Geometry check sheet. Reference: the model listing, model coordinates, mm. Coordinates: 2 decimals unless noted, no trailing zeros. Loops run counter-clockwise (first coordinate to the right, second up) from the corner with the lowest first, then second, coordinate; pieces in that order, holes last. Notation, with made-up numbers: M 27,27 L 39,27 A14 ccw 39,35 Z; hole C 25,53.5 d3. An arc over 180 degrees is marked long. Use CSV: the item, a comma, the result in double quotes.
```python
from build123d import *

# Parameters (mm, degrees)
SKETCH1_R           = 7
BOSS_EXTRUDE1_DEPTH = 5
SKETCH2_R           = 7.5
CUT_EXTRUDE1_DEPTH  = 10


with BuildPart() as part:
    # Sketch1 → Boss-Extrude1 (new body)
    with BuildSketch(Plane(origin=(0, 0, 0), x_dir=(1, 0, 0), z_dir=(0, 1, 0))):
        with BuildLine():
            Line((-415.542365302, 422.631578947), (-351.296475424, 422.631578947))
            Line((-351.296475424, 422.631578947), (-351.296475424, 222.631578947))
            Line((-351.296475424, 222.631578947), (-415.542365302, 222.631578947))
            Line((-415.542365302, 222.631578947), (-449.708642176, 172.131578947))
            Line((-449.708642176, 172.131578947), (-449.708642176, 121.631578947))
            ThreePointArc((-449.708642176, 121.631578947), (-452.637574364, 114.560511136), (-459.708642176, 111.631578947))
            Line((-459.708642176, 111.631578947), (-479.708642176, 111.631578947))
            ThreePointArc((-479.708642176, 111.631578947), (-486.779709988, 114.560511136), (-489.708642176, 121.631578947))
            Line((-489.708642176, 121.631578947), (-489.708642176, 172.131578947))
            Line((-489.708642176, 172.131578947), (-524.868977384, 222.631578947))
            Line((-524.868977384, 222.631578947), (-691.296475424, 222.631578947))
            Line((-691.296475424, 222.631578947), (-691.296475424, 142.631578947))
            Line((-691.296475424, 142.631578947), (-1821.296475424, 142.631578947))
            Line((-1821.296475424, 142.631578947), (-1821.296475424, 502.631578947))
            Line((-1821.296475424, 502.631578947), (-691.296475424, 502.631578947))
            Line((-691.296475424, 502.631578947), (-691.296475424, 422.631578947))
            Line((-691.296475424, 422.631578947), (-524.868977384, 422.631578947))
            Line((-524.868977384, 422.631578947), (-489.708642176, 473.131578947))
            Line((-489.708642176, 473.131578947), (-489.708642176, 523.631578947))
            ThreePointArc((-489.708642176, 523.631578947), (-486.779709988, 530.702646759), (-479.708642176, 533.631578947))
            Line((-479.708642176, 533.631578947), (-459.708642176, 533.631578947))
            ThreePointArc((-459.708642176, 533.631578947), (-452.637574364, 530.702646759), (-449.708642176, 523.631578947))
            Line((-449.708642176, 523.631578947), (-449.708642176, 473.131578947))
            Line((-449.708642176, 473.131578947), (-415.542365302, 422.631578947))
        make_face()
        with Locations((-469.708642176, 492.631578947)):
            Circle(SKETCH1_R, mode=Mode.SUBTRACT)
        with Locations((-469.708642176, 152.631578947)):
            Circle(SKETCH1_R, mode=Mode.SUBTRACT)
    extrude(amount=BOSS_EXTRUDE1_DEPTH)

    # Sketch2 → Cut-Extrude1 (cut)
    with BuildSketch(Plane(origin=(0, 5, 0), x_dir=(1, 0, 0), z_dir=(0, 1, 0))):
        with Locations((-1597.770206395, 392.549644623)):
            Circle(SKETCH2_R)
        with Locations((-1597.770206395, 240.60770245)):
            Circle(SKETCH2_R)
    extrude(amount=-CUT_EXTRUDE1_DEPTH, mode=Mode.SUBTRACT)


solid = part.part
```
1. Section check D-D, the plane z = -205.5. Record the cut outline in (x, y), plus the area to 3 significant figures.
The answers:
outline,"M -1821.3,0 L -691.3,0 L -691.3,5 L -1821.3,5 Z; M -512.94,0 L -427.13,0 L -427.13,5 L -512.94,5 Z"
area,"6,080 mm^2"
2. Gauge pin test, flat ends, axial feed: P1, Ø1.5, axis at x = -1157, y = 2, coming from the -Z side; P2, Ø11, axis at x = -469.71, z = -152.63, coming from the +Y side; P3, Ø3, axis at x = -528, y = 3.5, coming from the -Z side; P4, Ø2.5, axis at y = 2.5, z = -154, coming from the +X side. Record the tip position at first contact, or that the pin passes through.
The answers:
P1,"z = -502.63"
P2,"through"
P3,"z = -422.63"
P4,"x = -449.71"
3. Section check A-A, the plane z = -454.5. Record the cut outline in (x, y), plus the area to 3 significant figures.
The answers:
outline,"M -1821.3,0 L -691.3,0 L -691.3,5 L -1821.3,5 Z; M -502.68,0 L -437.1,0 L -437.1,5 L -502.68,5 Z"
area,"5,980 mm^2"
4. Thickness scan on line 1 (Z direction, x = -1700, y = 2.7); line 2 (Z direction, x = -571.5, y = 4.3); line 3 (X direction, y = 3.7, z = -438.5). Record the ranges inside material, lowest first. Write a range as [from, to].
The answers:
line 1,"[-502.63, -142.63]"
line 2,"[-422.63, -222.63]"
line 3,"[-1821.3, -691.3], [-513.82, -426.28]"
5. Release check for a two-part mould opening along X. For faces 1 (the flat face through (-507.535, 2.465, -447.528)), 2 (the flat face through (-1076, 0, -326)), 3 (the flat face through (-432.865, 2.465, -448.235)), 4 (the flat face through (-507.043, 2.465, -197.028)) record: +X half, -X half, draft (parallel to the pull), parting line (faces both ways), or undercut.
The answers:
face 1,"undercut"
face 2,"draft"
face 3,"+X half"
face 4,"undercut"
6. Section check B-B, the plane y = 2.4. Record the cut outline in (x, z), plus the area to 3 significant figures.
The answers:
outline,"M -1821.3,-502.63 L -691.3,-502.63 L -691.3,-422.63 L -524.87,-422.63 L -489.71,-473.13 L -489.71,-523.63 A10 ccw -479.71,-533.63 L -459.71,-533.63 A10 ccw -449.71,-523.63 L -449.71,-473.13 L -415.54,-422.63 L -351.3,-422.63 L -351.3,-222.63 L -415.54,-222.63 L -449.71,-172.13 L -449.71,-121.63 A10 ccw -459.71,-111.63 L -479.71,-111.63 A10 ccw -489.71,-121.63 L -489.71,-172.13 L -524.87,-222.63 L -691.3,-222.63 L -691.3,-142.63 L -1821.3,-142.63 Z; hole C -1597.77,-392.55 d15; hole C -1597.77,-240.61 d15; hole C -469.71,-492.63 d14; hole C -469.71,-152.63 d14"
area,"486,000 mm^2"
7. Section check C-C, the plane x = -1553. Record the cut outline in (y, z), plus the area to 3 significant figures.
The answers:
outline,"M 0,-502.63 L 5,-502.63 L 5,-142.63 L 0,-142.63 Z"
area,"1,800 mm^2"
